Model file for the job. Use its own axes, mm. Face numbers are marked on the shaded views. A direction names the side the tool comes from. Round coordinates to 2 decimals unless told otherwise and drop trailing zeros. Order: outer loops, then holes, each group sorted by start corner. A loop starts at its lowest first (then second) coordinate and runs counter-clockwise, first axis right, second up. Notation, with made-up numbers: (25, -20) -> (41, -20) arc R4 cw to (41, -16) -> close; hole circle Ø1 at (56, 85.5). An arc over 180 degrees is marked (long way). Use CSV: the item, a comma, the result in double quotes.
```python
from build123d import *

# Parameters (mm, degrees)
SKETCH1_R                = 15
BOSS_EXTRUDE1_DEPTH      = 80
SKETCH2_R                = 15
BOSS_EXTRUDE2_DEPTH      = 20
BOSS_EXTRUDE2_DRAFT      = -60
SKETCH3_R                = 125
BOSS_EXTRUDE5_DEPTH      = 30
BOSS_EXTRUDE5_DRAFT      = -30
SKETCH6_R                = 125
SKETCH6_R_2              = 115
BOSS_EXTRUDE6_DEPTH      = 10
SKETCH7_R                = 142.320508076
BOSS_EXTRUDE7_DEPTH      = 20
SKETCH9_R                = 142.320508076
BOSS_EXTRUDE8_DEPTH      = 30
BOSS_EXTRUDE8_TAPER      = 30
FILLET1_R                = 60
FILLET3_R                = 70
FILLET4_R                = 30
BOSS_EXTRUDE9_DEPTH      = 20
BOSS_EXTRUDE9_DEPTH_BACK = 305
SKETCH10_R               = 9.5


with BuildPart() as part:
    # Sketch1 → Boss-Extrude1 (new body)
    with BuildSketch(Plane.XY):
        Circle(SKETCH1_R)
    extrude(amount=BOSS_EXTRUDE1_DEPTH)


with BuildPart() as boss_extrude2_tool:
    # Sketch2 → Boss-Extrude2 (with draft: the straight prism first)
    with BuildSketch(Plane(origin=(0, 0, 0), x_dir=(-1, 0, 0), z_dir=(0, 0, -1))):
        Circle(SKETCH2_R)
    extrude(amount=BOSS_EXTRUDE2_DEPTH)
    # Boss-Extrude2: the draft: its side faces are tilted about the plane it starts from
    boss_extrude2_sides = [boss_extrude2_tool.faces().sort_by_distance(p)[0] for p in [
        (15, 0, -10),
    ]]
    draft(boss_extrude2_sides, Plane(origin=(0, 0, 0), x_dir=(-1, 0, 0), z_dir=(0, 0, -1)), BOSS_EXTRUDE2_DRAFT)


with BuildPart() as part_1:
    add(part.part)

    # Boss-Extrude2: add boss_extrude2_tool
    add(boss_extrude2_tool.part)


with BuildPart() as boss_extrude5_tool:
    # Sketch3 → Boss-Extrude5 (with draft: the straight prism first)
    with BuildSketch(Plane(origin=(0, 0, -20), x_dir=(-1, 0, 0), z_dir=(0, 0, -1))):
        Circle(SKETCH3_R)
    extrude(amount=BOSS_EXTRUDE5_DEPTH)
    # Boss-Extrude5: the draft: its side faces are tilted about the plane it starts from
    boss_extrude5_sides = [boss_extrude5_tool.faces().sort_by_distance(p)[0] for p in [
        (125, 0, -35),
    ]]
    draft(boss_extrude5_sides, Plane(origin=(0, 0, -20), x_dir=(-1, 0, 0), z_dir=(0, 0, -1)), BOSS_EXTRUDE5_DRAFT)


with BuildPart() as part_2:
    add(part_1.part)

    # Boss-Extrude5: add boss_extrude5_tool
    add(boss_extrude5_tool.part)

    # Sketch6 → Boss-Extrude6 (add)
    with BuildSketch(Plane.XY.offset(-20)):
        Circle(SKETCH6_R)
        Circle(SKETCH6_R_2, mode=Mode.SUBTRACT)
    extrude(amount=BOSS_EXTRUDE6_DEPTH)

    # Sketch7 → Boss-Extrude7 (add)
    with BuildSketch(Plane(origin=(0, 0, -50), x_dir=(-1, 0, 0), z_dir=(0, 0, -1))):
        Circle(SKETCH7_R)
    extrude(amount=BOSS_EXTRUDE7_DEPTH)

    # Sketch9 → Boss-Extrude8 (add)
    with BuildSketch(Plane(origin=(0, 0, -70), x_dir=(-1, 0, 0), z_dir=(0, 0, -1))):
        Circle(SKETCH9_R)
    extrude(amount=BOSS_EXTRUDE8_DEPTH, taper=BOSS_EXTRUDE8_TAPER)

    # Fillet1
    fillet1_edges = [part_2.edges().sort_by_distance(p)[0] for p in [
        (125, 0, -100),
    ]]
    fillet(fillet1_edges, radius=FILLET1_R - 0.0001)  # a hair under: the kernel refuses the full size

    # Fillet3
    fillet3_edges = [part_2.edges().sort_by_distance(p)[0] for p in [
        (142.320508076, 0, -50),
    ]]
    fillet(fillet3_edges, radius=FILLET3_R)

    # Fillet4
    fillet4_edges = [part_2.edges().sort_by_distance(p)[0] for p in [
        (0, -125, -20),
    ]]
    fillet(fillet4_edges, radius=FILLET4_R)

    # Sketch10 → Boss-Extrude9 (add, two sides: drawn at the far end of the back side and taken through both)
    with BuildSketch(Plane.ZY.offset(142.320508076).offset(-BOSS_EXTRUDE9_DEPTH_BACK)):
        with Locations((-54.490163429, 0)):
            Circle(SKETCH10_R)
    extrude(amount=BOSS_EXTRUDE9_DEPTH + BOSS_EXTRUDE9_DEPTH_BACK)


solid = part_2.part
```
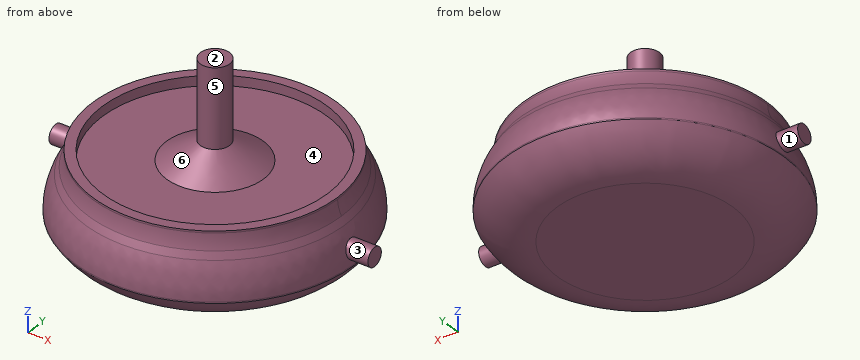
Q1. Cut at A-A (z = 62). Give the cut face in (x, y).
From the geometry:
outline,"circle Ø30 at (0, 0)"
Q2. Which spindle directions (+Z, -Z, +X, -X, +Y, -Y) get a long thin tool onto all of the face, cutting with end or side? Do the marked faces 1 and 2. Say none if no direction does.
From the geometry:
face 1,"-X"
face 2,"+Z, +X, -X, +Y, -Y"
Q3. Pin check, flat tips, straight feed: pin 1 (3 mm diameter, centred on y = -9.5, z = -71, fed in from +X); pin 2 (10 mm diameter, centred on y = -80.5, z = -77.5, fed in from +X); pin 3 (3 mm diameter, centred on x = -28, z = -42, fed in from -Y). Stop position of each tip, or through.
From the geometry:
pin 1,"stops at x = 142.07"
pin 2,"stops at x = 116.76"
pin 3,"stops at y = -134.8"
Q4. Probe line 1 along Y through (x, z) = (0, -16); line 2 along Y through (x, z) = (0, -15.5); line 3 along X through (y, z) = (-27, -19.5). List the from-to ranges inside material, lowest first.
From the geometry:
line 1,"y = -125.27 to -115, -42.71 to 42.71, 115 to 125.27"
line 2,"y = -125.21 to -115, -41.85 to 41.85, 115 to 125.21"
line 3,"x = -123.03 to -111.79, -40.62 to 40.62, 111.79 to 123.03"
Q5. Mould opens along X. For the marked faces 3, 4, 5 and 6 say: +X half, -X half, draft (parallel to the pull), parting line (faces both ways), or undercut.
From the geometry:
face 3,"draft"
face 4,"undercut"
face 5,"parting line"
face 6,"undercut"
